Answer from the drawing. Dimensions are ordinates in mm from the lowest x, y and z of the part. Coordinates: 2 decimals unless noted, no trailing zeros. Write each loop counter-clockwise with the first axis right and the second up, starting at its lowest first coordinate (ties: lowest second). Pieces come first, ordered by that corner, then holes. Notation, with made-up numbers: (43, -24) -> (81, -24) arc R18 cw to (81, -17) -> close; hole circle Ø10 at (47.25, 82.25). An arc over 180 degrees is marked (long way). Return JSON: item names as keys, results as strings.
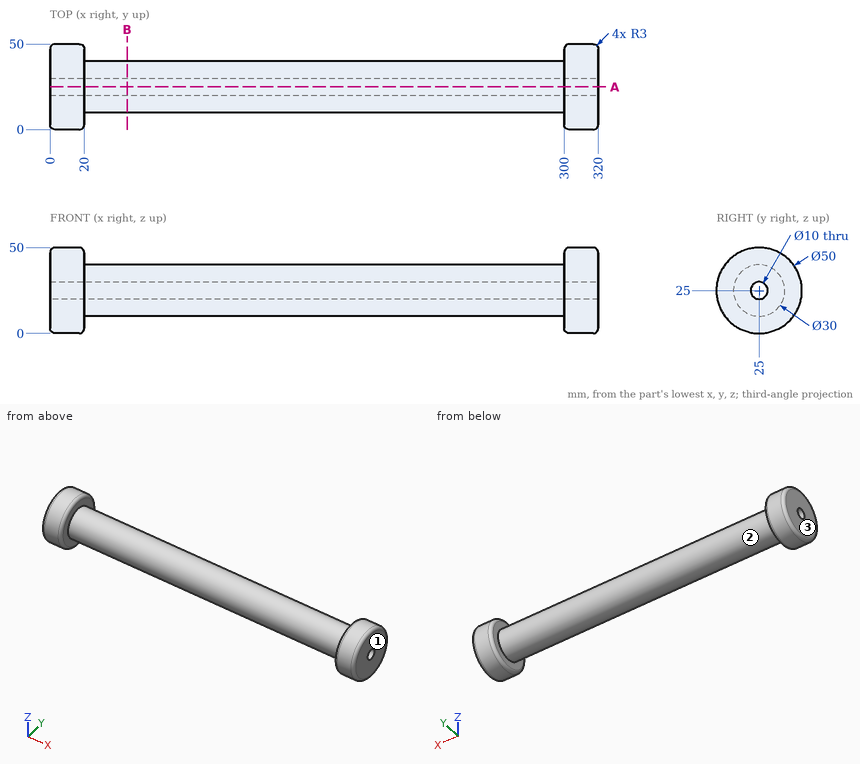
1. Consider L1, parallel to Y at x = 187, z = 25; L2, parallel to X at y = 9.5, z = 20; L3, parallel to Z at x = 67, y = 24. Determine where each line is inside the solid, lowest interval first.
Taken from the geometry:
{"L1": "y = 10 to 20, 30 to 40", "L2": "x = 0 to 20, 300 to 320", "L3": "z = 10.03 to 20.1, 29.9 to 39.97"}
2. The part is cut by section A-A (y = 25). Determine the outline of the cut face in (x, z).
Taken from the geometry:
{"outline": "(0, 3) arc R3 ccw to (3, 0) -> (17, 0) arc R3 ccw to (20, 3) -> (20, 10) -> (300, 10) -> (300, 3) arc R3 ccw to (303, 0) -> (317, 0) arc R3 ccw to (320, 3) -> (320, 20) -> (0, 20) -> close; (0, 30) -> (320, 30) -> (320, 47) arc R3 ccw to (317, 50) -> (303, 50) arc R3 ccw to (300, 47) -> (300, 40) -> (20, 40) -> (20, 47) arc R3 ccw to (17, 50) -> (3, 50) arc R3 ccw to (0, 47) -> close"}
3. The part is cut by section B-B (x = 45). Determine the outline of the cut face in (y, z), then the cut area to 3 significant figures.
Taken from the geometry:
{"outline": "circle Ø30 at (25, 25); hole circle Ø10 at (25, 25)", "area": "628 mm2"}
4. For a pull along X with two mould halves and no side action, classify the marked faces 1, 2 and 3 as +X half, -X half, draft (parallel to the pull), parting line (faces both ways), or undercut.
Taken from the geometry:
{"face 1": "+X half", "face 2": "undercut", "face 3": "-X half"}
5. Flat-ended cylindrical pins translate along their axes: pin 1 Ø12 at (x, y) = (133, 17) entering from -Z; pin 2 Ø1 at (y, z) = (28, 28) entering from +X; pin 3 Ø6 at (x, y) = (108.5, 26.5) entering from -Z; pin 4 Ø1.5 at (x, z) = (33, 34) entering from +Y. Find the tip coordinate at first contact, or state that the pin passes through.
Taken from the geometry:
{"pin 1": "stops at z = 10.13", "pin 2": "passes through", "pin 3": "stops at z = 10", "pin 4": "stops at y = 37.53"}
